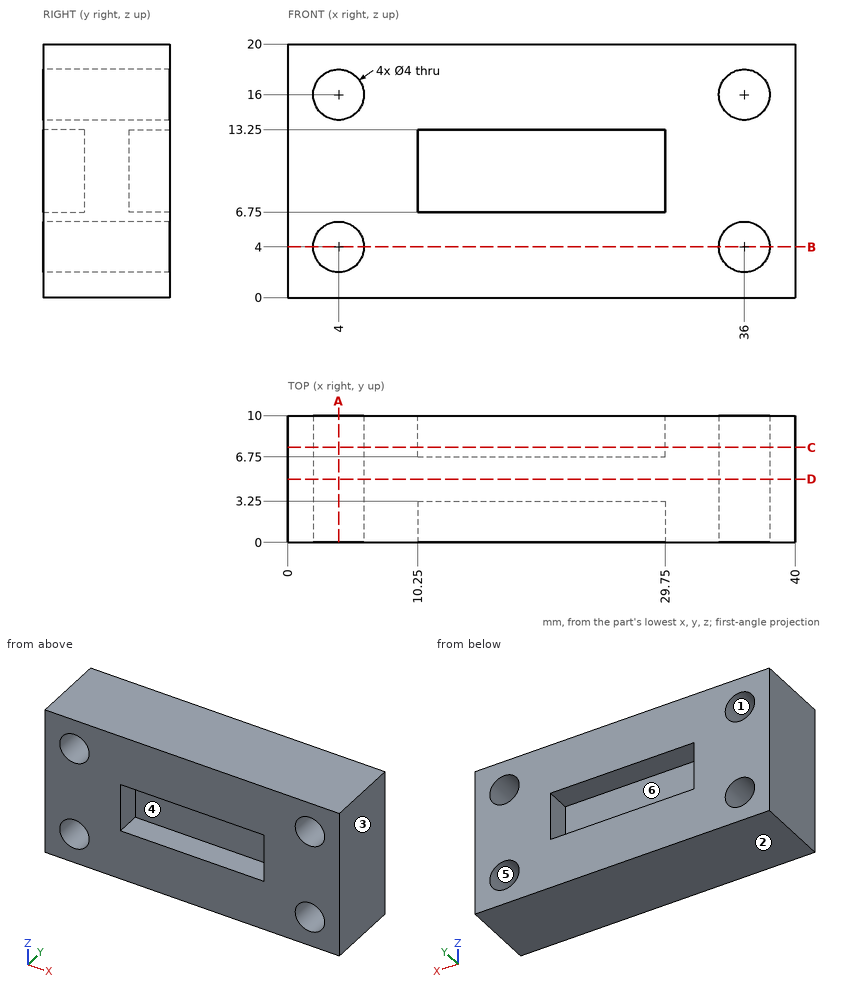
Check sheet for the drawn part. Datum: minimum x, y, z corner. Units: mm. A direction names the side the tool comes from. Coordinates: 2 decimals unless noted, no trailing zeros. Order: outer loops, then holes, each group sorted by start corner. A loop starts at its lowest first (then second) coordinate and runs counter-clockwise, first axis right, second up. Notation, with made-up numbers: M -4,-16.75 L 49,-16.75 A20 ccw 49,19.25 Z; hole C -26,2.25 d9. An arc over 180 degrees is marked long. One line per question, with ' | ' between items. Start each with the question number.
Item 1: Sectioned sample at D-D on y = 5. Record the cut outline in (x, z), and give its area (3 significant figures).
Item 2: Mould release check, pull along X, two halves, no side actions. Record for the marked faces 1, 2 and 3: pulls with the +X half, pulls with the -X half, needs draft (parallel to the pull), parting line crosses it, or undercut.
Item 3: Sectioned sample at B-B on z = 4. Record the cut outline in (x, y).
Item 4: Gauge pin test, flat ends, axial feed: P1, Ø3, axis at x = 4, z = 16, coming from the -Y side; P2, Ø4, axis at x = 24.5, z = 9, coming from the +Y side; P3, Ø5, axis at x = 18, z = 9.5, coming from the -Y side. Record the tip position at first contact, or that the pin passes through.
Item 5: Access from +Z, -Z, +X, -X, +Y, -Y to the whole of each face (thin tool, end or side, straight path). Record for the marked faces 4, 5 and 6.
Item 6: Sectioned sample at C-C on y = 7.5. Record the cut outline in (x, z), and give its area (3 significant figures).
Item 7: Sectioned sample at A-A on x = 4. Record the cut outline in (y, z), and give its area (3 significant figures).
Item 8: Material ranges on line 1 (X direction, y = 5.25, z = 4); line 2 (X direction, y = 7.25, z = 11.5); line 3 (X direction, y = 9.5, z = 2.5), recorded low to high.
Answer below:
1) outline: M 0,0 L 40,0 L 40,20 L 0,20 Z; hole C 4,4 d4; hole C 4,16 d4; hole C 36,4 d4; hole C 36,16 d4 | area: 750 mm^2
2) face 1: undercut | face 2: needs draft | face 3: pulls with the +X half
3) outline: M 0,0 L 2,0 L 2,10 L 0,10 Z; M 6,0 L 34,0 L 34,10 L 6,10 Z; M 38,0 L 40,0 L 40,10 L 38,10 Z
4) P1: passes through | P2: stops at y = 6.75 | P3: stops at y = 3.25
5) face 4: -Y | face 5: +Y, -Y | face 6: +Y
6) outline: M 0,0 L 40,0 L 40,20 L 0,20 Z; hole C 4,4 d4; hole C 4,16 d4; hole M 10.25,6.75 L 29.75,6.75 L 29.75,13.25 L 10.25,13.25 Z; hole C 36,4 d4; hole C 36,16 d4 | area: 623 mm^2
7) outline: M 0,0 L 10,0 L 10,2 L 0,2 Z; M 0,6 L 10,6 L 10,14 L 0,14 Z; M 0,18 L 10,18 L 10,20 L 0,20 Z | area: 120 mm^2
8) line 1: x = 0 to 2, 6 to 34, 38 to 40 | line 2: x = 0 to 10.25, 29.75 to 40 | line 3: x = 0 to 2.68, 5.32 to 34.68, 37.32 to 40
